Study the drawing (mm; zero at the part's minimum x, y, z) and answer. Coordinates: 2 decimals unless noted, no trailing zeros. Order: outer loops, then holes, each group sorted by start corner. A loop starts at its lowest first (then second) coordinate and runs counter-clockwise, first axis right, second up.
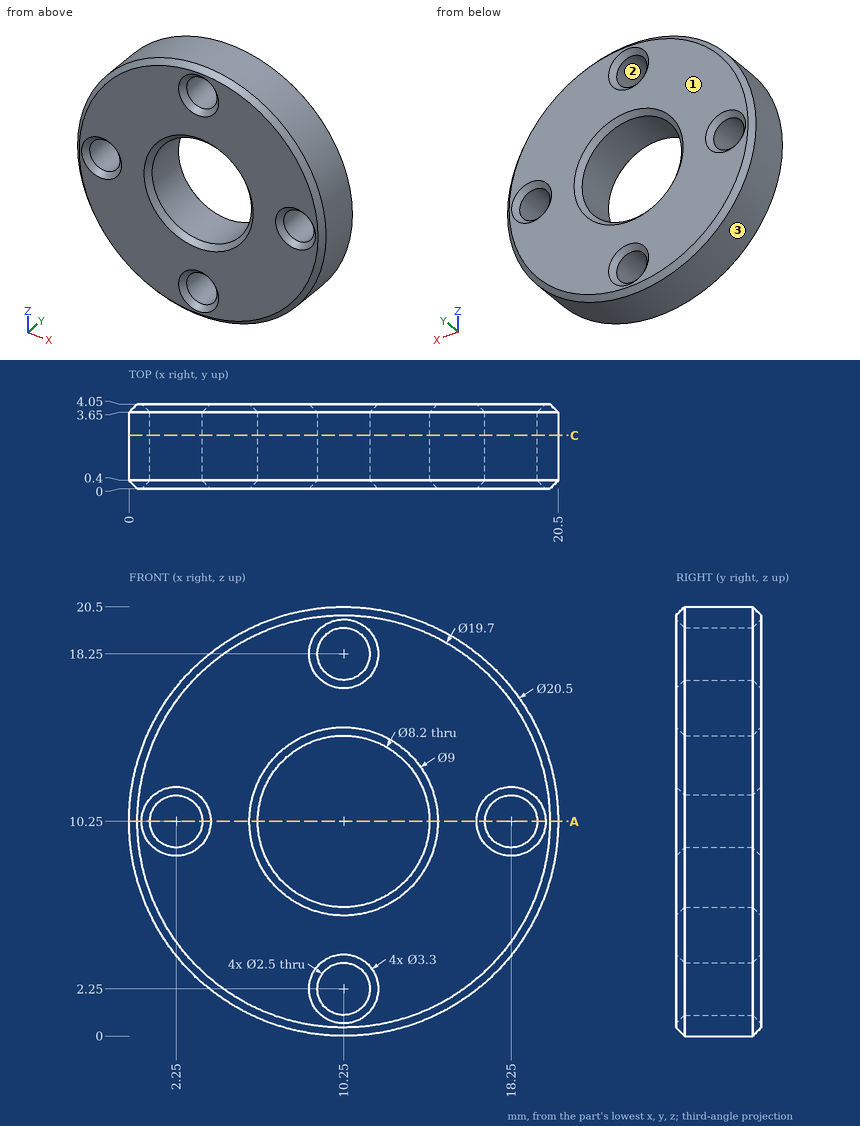
1) Determine the mould class of the marked faces 1, 2 and 3 for opening direction Z: pulls with the +Z half, pulls with the -Z half, needs draft (parallel to the pull), parting line crosses it, or undercut.
A:
face 1: needs draft
face 2: undercut
face 3: parting line crosses it
2) Flat-ended cylindrical pins translate along their axes: pin 1 Ø2 at (x, z) = (10.25, 2.25) entering from -Y; pin 2 Ø3 at (x, z) = (2.25, 10.25) entering from -Y; pin 3 Ø1.5 at (x, y) = (6, 0.5) entering from -Z; pin 4 Ø5 at (x, z) = (13, 6.5) entering from -Y. Find the tip coordinate at first contact, or state that the pin passes through.
A:
pin 1: passes through
pin 2: stops at y = 0.15
pin 3: stops at z = 0.62
pin 4: stops at y = 0
3) Straight lines are drawn through the part: line 1 (Z direction, x = 10.25, y = 2.7); line 2 (Z direction, x = 9.75, y = 0.85). For each, find the intervals that lie inside material, in ascending order.
A:
line 1: z = 0 to 1, 3.5 to 6.15, 14.35 to 17, 19.5 to 20.5
line 2: z = 0.01 to 1.1, 3.4 to 6.18, 14.32 to 17.1, 19.4 to 20.49
4) A cutting plane is placed at C-C, the plane y = 2.55. Determine the outline of the cut face in (x, z).
A:
outline: circle Ø20.5 at (10.25, 10.25); hole circle Ø2.5 at (2.25, 10.25); hole circle Ø8.2 at (10.25, 10.25); hole circle Ø2.5 at (10.25, 2.25); hole circle Ø2.5 at (10.25, 18.25); hole circle Ø2.5 at (18.25, 10.25)
5) A cutting plane is placed at A-A, the plane z = 10.25. State how many separate pieces and enclosed holes the cut face has, and give its area (3 significant figures).
A:
separate pieces: 4
enclosed holes: 0
area: 28.3 mm2
